```python
from build123d import *

# Parameters (mm, degrees)
SKETCH_1_R      = 15
EXTRUDE_1_DEPTH = 30
FILLET_1_R      = 1


with BuildPart() as part:
    # 草图1 → 凸台-拉伸1 (new body)
    with BuildSketch(Plane.XY):
        Circle(SKETCH_1_R)
    extrude(amount=EXTRUDE_1_DEPTH)

    # 圆角1
    fillet_1_edges = [part.edges().sort_by_distance(p)[0] for p in [
        (-15, 0, 0),
        (-15, 0, 30),
    ]]
    fillet(fillet_1_edges, radius=FILLET_1_R)

    # 草图2 → 切除-旋转1 (revolve, cut)
    with BuildSketch(Plane(origin=(0, 0, 0), x_dir=(1, 0, 0), z_dir=(0, 1, 0)), mode=Mode.PRIVATE) as cut_revolve_1_sk:
        with BuildLine():
            Line((0, 0), (3, 0))
            ThreePointArc((3, 0), (2.724744871, -0.866025404), (2, -1.414213562))
            ThreePointArc((2, -1.414213562), (1.642804036, -2.088628074), (1, -2.5))
            ThreePointArc((1, -2.5), (0.707106781, -1.792893219), (0, -1.5))
            Line((0, -1.5), (0, 0))
        make_face()
    revolve(cut_revolve_1_sk.sketch.rotate(Axis((0, 0, -2.778762471), (0, 0, 1)), 180), axis=Axis((0, 0, -2.778762471), (0, 0, 1)), mode=Mode.SUBTRACT)


solid = part.part
```
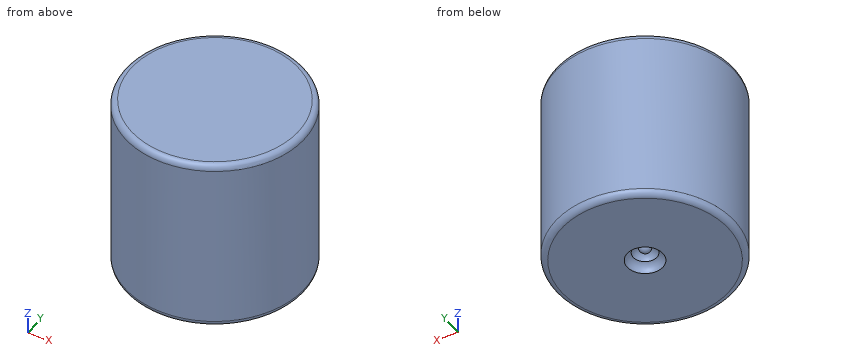
Input: part model. Units: mm. Frame: model coordinates. Coordinates: 2 decimals unless noted, no trailing zeros. Write each loop counter-clockwise with the first axis right and the second up, starting at its lowest first coordinate (ties: lowest second). Pieces come first, ordered by that corner, then holes. Notation, with made-up numbers: (57.25, 65.25) -> (103.25, 65.25) arc R26 ccw to (103.25, 91.25) -> close; hole circle Ø1 at (-2.75, -16.5). An arc over 180 degrees is marked (long way). Write each question's results on one line, items separated by ' | '.
Item 1: Pin query (flat end, axial travel): pin 1 Ø4 at (y, z) = (-11.5, 14) entering from +X; pin 2 Ø1 at (x, y) = (-1.5, 1.5) entering from -Z; pin 3 Ø8 at (y, z) = (-7, 26.5) entering from +X. Return the tip coordinate at first contact, or that it passes through.
Conclusion:
pin 1: stops at x = 11.61 | pin 2: stops at z = 1 | pin 3: stops at x = 14.7
Item 2: Material intervals for probe 1 along Y at (x, z) = (-11.75, 10); probe 2 along X at (y, z) = (3, 20.75); probe 3 along X at (y, z) = (-2.25, 5), sorted ascending.
Conclusion:
probe 1: y = -9.32 to 9.32 | probe 2: x = -14.7 to 14.7 | probe 3: x = -14.83 to 14.83
Item 3: Section query A-A on z = 9. Return loops of the section in (x, y).
Conclusion:
outline: circle Ø30 at (0, 0)
